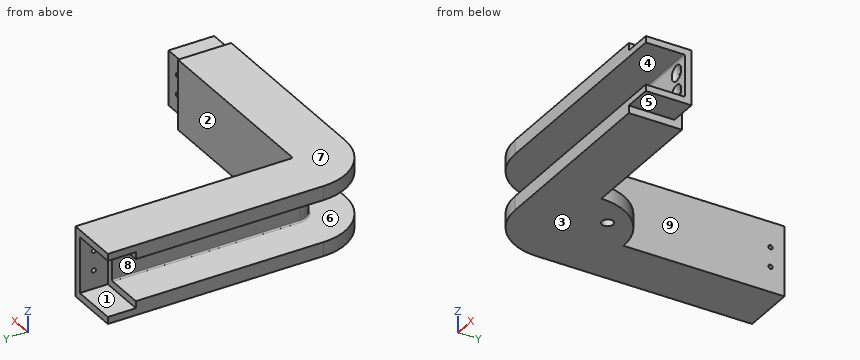
from build123d import *

# Parameters (mm, degrees)
BOSS_EXTRUDE2_START  = 12.7
BOSS_EXTRUDE2_DEPTH  = 12.7
BOSS_EXTRUDE3_DEPTH  = 12.7
SKETCH8_R            = 0.9525
CUT_EXTRUDE1_DEPTH   = 146.526980066
SKETCH9_R            = 0.9525
CUT_EXTRUDE2_DEPTH   = 152.345956246
SKETCH12_R           = 2.5527
BOSS_EXTRUDE10_DEPTH = 6.35


with BuildPart() as part:
    # Sweep1: sweep along a path in Sketch4
    with BuildLine(Plane.XY) as sweep1_path:
        Line((0, 0), (0, -85.09))
        ThreePointArc((0, -85.09), (0.223184633, -85.628815367), (0.762, -85.852))
        Line((0.762, -85.852), (85.852, -85.852))
    # Sketch3 → Sweep1 (sweep)
    with BuildSketch(Plane(origin=(0, 0, 0), x_dir=(1, 0, 0), z_dir=(0, 1, 0))):
        with BuildLine():
            Line((0, 10.27500014), (-24.13, 10.27500014))
            Line((-24.13, 10.27500014), (-24.13, 3.92500014))
            Line((-24.13, 3.92500014), (-6.985, 3.92500014))
            ThreePointArc((-6.985, 3.92500014), (-6.535987194, 3.739012946), (-6.35, 3.29000014))
            Line((-6.35, 3.29000014), (-6.35, -14.48999986))
            ThreePointArc((-6.35, -14.48999986), (-6.535987194, -14.939012666), (-6.985, -15.12499986))
            Line((-6.985, -15.12499986), (-24.13, -15.12499986))
            Line((-24.13, -15.12499986), (-24.13, -21.47499986))
            Line((-24.13, -21.47499986), (0, -21.47499986))
            Line((0, -21.47499986), (0, 10.27500014))
        make_face()
    sweep(path=sweep1_path.line)

    # Sketch6 → Boss-Extrude2 (add)
    with BuildSketch(Plane(origin=(85.852, 0, 0), x_dir=(0, 0, -1), z_dir=(1, 0, 0)).offset(BOSS_EXTRUDE2_START)):
        with BuildLine():
            Line((-18.04599986, -89.281), (6.84600014, -89.281))
            Line((6.84600014, -89.281), (6.84600014, -109.982))
            Line((6.84600014, -109.982), (3.92500014, -109.982))
            Line((3.92500014, -109.982), (3.92500014, -92.837))
            ThreePointArc((3.92500014, -92.837), (3.739012946, -92.387987194), (3.29000014, -92.202))
            Line((3.29000014, -92.202), (-14.48999986, -92.202))
            ThreePointArc((-14.48999986, -92.202), (-14.939012666, -92.387987194), (-15.12499986, -92.837))
            Line((-15.12499986, -92.837), (-15.12499986, -109.982))
            Line((-15.12499986, -109.982), (-18.04599986, -109.982))
            Line((-18.04599986, -109.982), (-18.04599986, -89.281))
        make_face()
    extrude(amount=-BOSS_EXTRUDE2_DEPTH)

    # Sketch7 → Boss-Extrude3 (add)
    with BuildSketch(Plane(origin=(0, 0, 0), x_dir=(1, 0, 0), z_dir=(0, 1, 0))):
        Polygon((-24.13, 7.10000014), (-24.13, 10.27500014), (0, 10.27500014), (0, -21.47499986), (-24.13, -21.47499986), (-24.13, -18.29999986), (-3.175, -18.29999986), (-3.175, 7.10000014), align=None)
    extrude(amount=BOSS_EXTRUDE3_DEPTH)

    # Sketch8 → Cut-Extrude1 (cut, through all)
    with BuildSketch(Plane.XZ.offset(92.202)):
        with Locations(Location((92.202, 10.04499986, 0), (0, 0, 270))):
            Circle(SKETCH8_R)
        with Locations(Location((92.202, 1.15499986, 0), (0, 0, 270))):
            Circle(SKETCH8_R)
    extrude(amount=-CUT_EXTRUDE1_DEPTH, mode=Mode.SUBTRACT)

    # Sketch9 → Cut-Extrude2 (cut, through all)
    with BuildSketch(Plane.ZY.offset(3.175)):
        with Locations((1.15499986, 6.35)):
            Circle(SKETCH9_R)
        with Locations((10.04499986, 6.35)):
            Circle(SKETCH9_R)
    extrude(amount=-CUT_EXTRUDE2_DEPTH, mode=Mode.SUBTRACT)

    # Sketch12 → Boss-Extrude10 (add)
    with BuildSketch(Plane.XY.offset(-10.27500014)):
        with BuildLine():
            Line((0, -60.229795925), (0, -85.09))
            ThreePointArc((0, -85.09), (0.223184633, -85.628815367), (0.762, -85.852))
            Line((0.762, -85.852), (25.622204075, -85.852))
            ThreePointArc((25.622204075, -85.852), (18.183696875, -67.668303125), (0, -60.229795925))
        make_face()
        with Locations((11.43, -74.422)):
            Circle(SKETCH12_R, mode=Mode.SUBTRACT)
    extrude(amount=BOSS_EXTRUDE10_DEPTH)

    # Sketch14 → CSK for _6 Flat Head Machine Screw _100 (revolve, cut)
    with BuildSketch(Plane(origin=(92.202, -92.202, 1.15499986), x_dir=(0, 0, -1), z_dir=(1, 0, 0))):
        Polygon((0, 0), (0, 2.410824014), (1.89865, 1.27), (1.89865, 1.380025208), (3.5433, 0), align=None)
    revolve(axis=Axis((92.202, -98.552, 1.15499986), (0, 1, 0)), mode=Mode.SUBTRACT)

    # Sketch16 → CSK for _6 Flat Head Machine Screw _ 2 (revolve, cut)
    with BuildSketch(Plane(origin=(92.202, -92.202, 10.04499986), x_dir=(0, 0, -1), z_dir=(1, 0, 0))):
        Polygon((0, 0), (0, 2.410824014), (1.89865, 1.27), (1.89865, 1.380025208), (3.5433, 0), align=None)
    revolve(axis=Axis((92.202, -98.552, 10.04499986), (0, 1, 0)), mode=Mode.SUBTRACT)


solid = part.part
Can you work these out from the model? Positions are in its coordinate system, mm. Face numbers are marked on the shaded views. A direction names the side the tool comes from. Coordinates: 2 decimals unless noted, no trailing zeros. Loops run counter-clockwise (first coordinate to the right, second up) from the corner with the lowest first, then second, coordinate; pieces in that order, holes last. Notation, with made-up numbers: (74, -15.5) - (121, -15.5) arc R35 ccw to (121, 17.5) - close; hole circle Ø11 at (-1.75, 11). An arc over 180 degrees is marked (long way). Answer as a JSON object with one key per item and string values. Group by question number.
Item 1: On a 3-axis mill with a long thin cutter (end or side, diameter ignored), from which of +Z, -Z, +X, -X, +Y, -Y can I reach the whole of each face in a straight line? I mean the marked faces 1, 2, 3, 4 and 5. Say none if no direction works.
Item 2: For pin 1 (2.5 mm diameter, centred on x = 92.202, z = 1.155, fed in from +Y); pin 2 (1.5 mm diameter, centred on x = 11.5, z = 11, fed in from +Y); pin 3 (3 mm diameter, centred on y = 6.35, z = 1.155, fed in from -X) (3 decimals); pin 4 (1.7 mm diameter, centred on y = 6.35, z = 10.045, fed in from +X), each with a flat end and sliding along its axis, tell me the tip position at first contact or that it passes through.
Item 3: If we section it at D-D (y = -94.5): List the corners of the cut face in (x, z) for me (3 decimals), plus the area to 3 significant figures.
Item 4: If we section it at A-A (y = 2): List the corners of the cut face in (x, z) for me (3 decimals).
Item 5: If we section it at C-C (x = 49.5): List the corners of the cut face in (y, z) for me (3 decimals), plus the area to 3 significant figures.
Item 6: If we section it at B-B (x = -16): List the corners of the cut face in (y, z) for me (3 decimals), plus the area to 4 significant figures.
Item 7: If we mould it in two halves opening along Z, with no side actions, what happens to the marked faces 6, 7, 8 and 9? For each: released by +Z, released by -Z, zero draft, split by the parting line, or undercut.
Item 8: If I drill on L1, parallel to Z at x = -14, y = -60.5 (3 decimals); L2, parallel to X at y = -57.5, z = -4; L3, parallel to X at y = -7, z = 12, over which ranges is the centre line in solid material (lowest first)? Write a range as from..to.
Returned:
{
 "1": {"face 1": "-X, +Y", "face 2": "+Z, +X, +Y", "face 3": "-Z, +X, -X, +Y, -Y", "face 4": "-X, -Y", "face 5": "-Z, +X, +Y, -Y"},
 "2": {"pin 1": "stops at y = -89.28", "pin 2": "stops at y = -85.85", "pin 3": "stops at x = -3.175", "pin 4": "passes through"},
 "3": {"outline": "(-22.283, -10.275) - (85.852, -10.275) - (85.852, -6.846) - (98.552, -6.846) - (98.552, -3.925) - (-22.283, -3.925) - close; (-22.283, 15.125) - (98.552, 15.125) - (98.552, 18.046) - (85.852, 18.046) - (85.852, 21.475) - (-22.283, 21.475) - close", "area": "1,450 mm²"},
 "4": {"outline": "(-24.13, -10.275) - (0, -10.275) - (0, 21.475) - (-24.13, 21.475) - (-24.13, 18.3) - (-3.175, 18.3) - (-3.175, -7.1) - (-24.13, -7.1) - close"},
 "5": {"outline": "(-109.982, -10.275) - (-85.852, -10.275) - (-85.852, 21.475) - (-109.982, 21.475) - (-109.982, 15.125) - (-92.837, 15.125) arc R0.635 cw to (-92.202, 14.49) - (-92.202, -3.29) arc R0.635 cw to (-92.837, -3.925) - (-109.982, -3.925) - close", "area": "428 mm²"},
 "6": {"outline": "(-103.492, -10.275) - (12.7, -10.275) - (12.7, -7.1) - (0, -7.1) - (0, -3.925) - (-103.492, -3.925) - close; (-103.492, 15.125) - (0, 15.125) - (0, 18.3) - (12.7, 18.3) - (12.7, 21.475) - (-103.492, 21.475) - close", "area": "1,395 mm²"},
 "7": {"face 6": "undercut", "face 7": "released by +Z", "face 8": "undercut", "face 9": "zero draft"},
 "8": {"L1": "z = -10.275..-3.925, 15.125..21.475", "L2": "x = -24.13..0", "L3": "x = -6.35..0"}
}
